```python
from build123d import *

# Parameters (mm, degrees)
DWIRE022_W       = 9.039794
DWIRE022_H       = 6.083538
EXTRUDE025_DEPTH = 6
DWIRE007_W       = 1.028705
DWIRE007_H       = 1.001781
EXTRUDE007_DEPTH = 9
ARRAY001_Y_COUNT = 20
ARRAY001_Y_PITCH = 2
DWIRE016_W       = 0.7
DWIRE016_H       = 38.839707
EXTRUDE019_DEPTH = 9
DWIRE021_W       = 3.095468
DWIRE021_H       = 4.884044
EXTRUDE024_DEPTH = 6


with BuildPart() as obj1:
    # DWire022 → Extrude025 (new body)
    with BuildSketch(Plane.XY):
        with Locations((-2.105889, 36.976721)):
            Rectangle(DWIRE022_W, DWIRE022_H)
    extrude(amount=EXTRUDE025_DEPTH)


with BuildPart() as obj1_1:
    # Extrude025 placement: moved
    add(obj1.part.moved(Location((0, 0, 6))))


with BuildPart() as obj2:
    # DWire007 → Extrude007 (new body)
    with BuildSketch(Plane.XY):
        with Locations((0.514352, 0.500891)):
            Rectangle(DWIRE007_W, DWIRE007_H)
    extrude(amount=EXTRUDE007_DEPTH)


with BuildPart() as obj2_1:
    # Extrude007 placement: moved
    add(obj2.part.moved(Location((0, 0, 6))))

    # Array001 Y: obj2 ×20


with BuildPart() as obj2_2:
    add(obj2_1.part)
    with Locations(*[(0, i * ARRAY001_Y_PITCH, 0) for i in range(1, ARRAY001_Y_COUNT)]):
        add(obj2_1.part)


with BuildPart() as obj3:
    # DWire016 → Extrude019 (new body)
    with BuildSketch(Plane.XY):
        with Locations((-0.05, 19.419853)):
            Rectangle(DWIRE016_W, DWIRE016_H)
    extrude(amount=EXTRUDE019_DEPTH)


with BuildPart() as obj3_1:
    # Extrude019 placement: moved
    add(obj3.part.moved(Location((0, 0, 6))))

    # Fusion002: union obj2
    add(obj2_2.part)


with BuildPart() as obj4:
    # Clone005 base: copy of obj3
    add(obj3_1.part)


with BuildPart() as part_mirroring004:
    # Part__Mirroring004: instance of obj4
    add(obj4.part.mirror(Plane(origin=(0, 0, 0), x_dir=(0, -1, 0), z_dir=(1, 0, 0))))


with BuildPart() as part_mirroring004_1:
    # Part__Mirroring004 placement: moved
    add(part_mirroring004.part.moved(Location((-3, 0, 0))))


with BuildPart() as extrude024:
    # DWire021 → Extrude024 (new body)
    with BuildSketch(Plane.XY):
        with Locations((-1.547734, 36.428072)):
            Rectangle(DWIRE021_W, DWIRE021_H)
    extrude(amount=EXTRUDE024_DEPTH)


with BuildPart() as extrude024_1:
    # Extrude024 placement: moved
    add(extrude024.part.moved(Location((0, 0, 6))))


with BuildPart() as obj5:
    # Fusion003 base: copy of obj3
    add(obj3_1.part)

    # Fusion003: union Part__Mirroring004, Extrude024
    add(part_mirroring004_1.part)
    add(extrude024_1.part)

    # Common: intersect obj1
    add(obj1_1.part, mode=Mode.INTERSECT)


solid = obj5.part
```
Model file for the job. Use its own axes, mm. A direction names the side the tool comes from. Coordinates: 2 decimals unless noted, no trailing zeros. Order: outer loops, then holes, each group sorted by start corner. A loop starts at its lowest first (then second) coordinate and runs counter-clockwise, first axis right, second up. Notation, with made-up numbers: (-34, 64.25) -> (-10, 64.25) arc R20 cw to (-10, 92.25) -> close; hole circle Ø7 at (53, -8.75). An arc over 180 degrees is marked (long way). Return JSON: item names as keys, results as strings.
Item 1: Slice it at A-A (x = -3.55). Write the cut outline in (y, z).
Model answer:
{"outline": "(34, 6) -> (35, 6) -> (35, 12) -> (34, 12) -> close; (36, 6) -> (37, 6) -> (37, 12) -> (36, 12) -> close; (38, 6) -> (39, 6) -> (39, 12) -> (38, 12) -> close"}
Item 2: Pin check, flat tips, straight feed: P1, Ø2, axis at x = -0.5, z = 10, coming from the -Y side; P2, Ø1.1, axis at x = -2, z = 9.5, coming from the -Y side; P3, Ø0.5, axis at y = 35.5, z = 10.5, coming from the -X side; P4, Ø0.5, axis at y = 35.5, z = 9, coming from the +X side. Stop position of each tip, or through.
Model answer:
{"P1": "stops at y = 33.93", "P2": "stops at y = 33.99", "P3": "stops at x = -3.3", "P4": "stops at x = 0.3"}
Item 3: 3-axis set-ups, long thin cutter, end or side, ignore diameter. For faces 1 (the face through (1.029, 34.5, 9)), 2 (the face through (0.3, 35.5, 9)), 3 (the face through (-2, 33.986, 9)): which of +Z, -Z, +X, -X, +Y, -Y reach the whole face in a straight line?
Model answer:
{"face 1": "+Z, -Z, +X, +Y, -Y", "face 2": "+Z, -Z, +X", "face 3": "+Z, -Z, -Y"}
Item 4: Slice it at C-C (y = 37.4). Write the cut outline in (x, z).
Model answer:
{"outline": "(-3.3, 6) -> (0.3, 6) -> (0.3, 12) -> (-3.3, 12) -> close"}
Item 5: Wall check: line 1 along Y through (x, z) = (0.4, 10.5); line 2 along X through (y, z) = (35.2, 7.75); line 3 along Y through (x, z) = (-1.8, 11.7). Give the ranges that are in metal, low to high. Write a range as from..to.
Model answer:
{"line 1": "y = 34..35, 36..37, 38..39", "line 2": "x = -3.3..0.3", "line 3": "y = 33.99..38.87"}
Item 6: Mould opens along Y. For faces 4 (the face through (-3.3, 37.5, 9)), 5 (the face through (-2, 37, 12)), 6 (the face through (-3.3, 35.5, 9)), 7 (the face through (-2, 38.87, 9)) say: pulls with the +Y half, pulls with the -Y half, needs draft (parallel to the pull), parting line crosses it, or undercut.
Model answer:
{"face 4": "undercut", "face 5": "needs draft", "face 6": "undercut", "face 7": "pulls with the +Y half"}
Item 7: Slice it at D-D (x = -0.15). Write the cut outline in (y, z), then the cut area to 3 significant figures.
Model answer:
{"outline": "(33.93, 6) -> (38.87, 6) -> (38.87, 12) -> (33.93, 12) -> close", "area": "29.6 mm²"}
